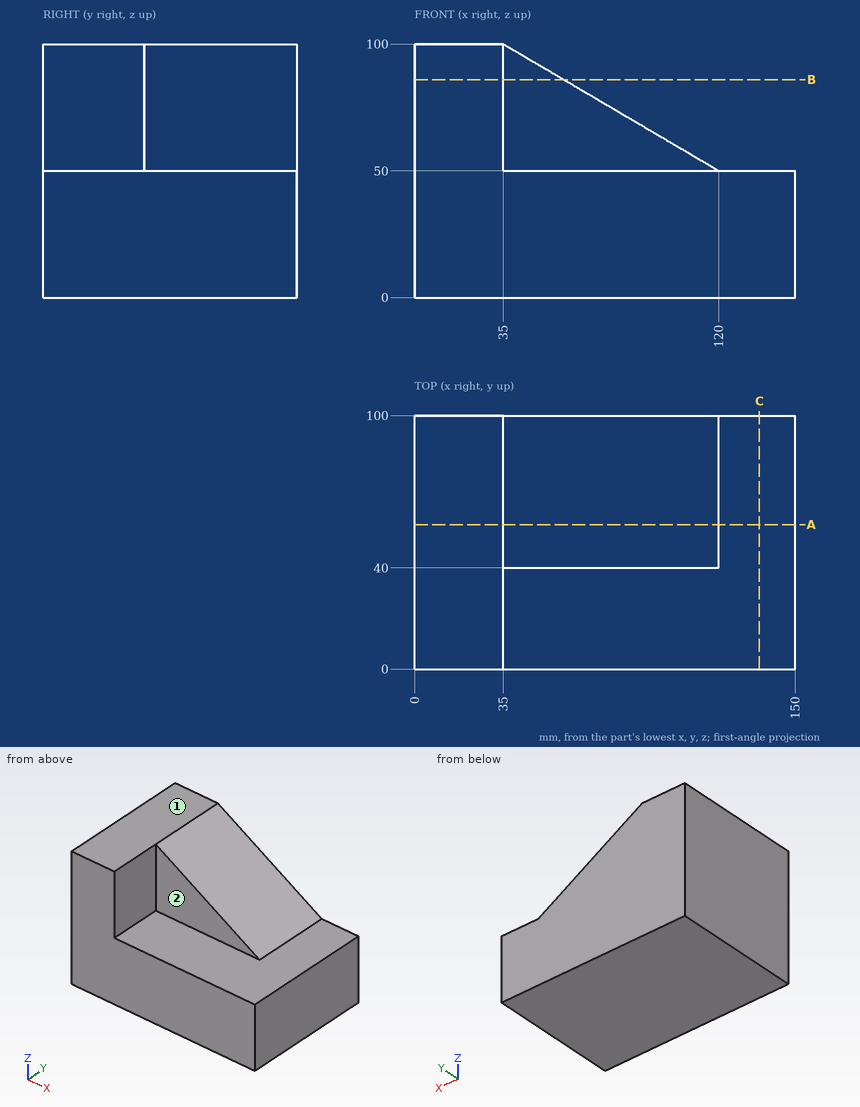
The drawing under review shows one solid part. Ordinate dimensions are in mm from its lowest x, y, z. A direction names the side the tool comes from. Round coordinates to 2 decimals unless told otherwise and drop trailing zeros. Loops run counter-clockwise (first coordinate to the right, second up) from the corner with the lowest first, then second, coordinate; pieces in that order, holes last. Notation, with made-up numbers: (-40, 71) -> (-25, 71) arc R15 ccw to (-25, 86) -> close; hole circle Ø9 at (-8.5, 25.25). An arc over 180 degrees is marked (long way). Answer in a Markdown table with one row per item.
1) Consider section C-C, the plane x = 136. Write out the cut boundary in (y, z), plus the area to 3 significant figures.
Taken from the geometry:
| item | result |
|---|---|
| outline | (0, 0) -> (100, 0) -> (100, 50) -> (0, 50) -> close |
| area | 5,000 mm² |
2) Wall thickness on line 1 along Z through (x, y) = (52.5, 37.5); line 2 along Y through (x, z) = (40, 78.5); line 3 along X through (y, z) = (12, 94.5): over which ranges is each line inside the solid? List them lowest first.
Taken from the geometry:
| item | result |
|---|---|
| line 1 | z = 0 to 50 |
| line 2 | y = 40 to 100 |
| line 3 | x = 0 to 35 |
3) Tool access review of the marked faces 1 and 2: name each direction out of +Z, -Z, +X, -X, +Y, -Y from which nothing blocks a thin tool from reaching the whole face with its end or side.
Taken from the geometry:
| item | result |
|---|---|
| face 1 | +Z, +X, -X, +Y, -Y |
| face 2 | +Z, +X, -Y |
4) Consider section B-B, the plane z = 86. Write out the cut boundary in (x, y).
Taken from the geometry:
| item | result |
|---|---|
| outline | (0, 0) -> (35, 0) -> (35, 40) -> (58.8, 40) -> (58.8, 100) -> (0, 100) -> close |
5) For pin 1 Ø1 at (x, y) = (123.5, 53.5) entering from -Z; pin 2 Ø12 at (y, z) = (11, 68) entering from +X; pin 3 Ø4 at (x, y) = (112.5, 78.5) entering from +Z; pin 4 Ø25 at (x, z) = (76, 64.5) entering from -Y, all flat-tipped, find the tip position at first contact; note any pin that passes through.
Taken from the geometry:
| item | result |
|---|---|
| pin 1 | stops at z = 0 |
| pin 2 | stops at x = 35 |
| pin 3 | stops at z = 55.59 |
| pin 4 | stops at y = 40 |
6) Consider section A-A, the plane y = 57. Write out the cut boundary in (x, z), plus the area to 3 significant figures.
Taken from the geometry:
| item | result |
|---|---|
| outline | (0, 0) -> (150, 0) -> (150, 50) -> (120, 50) -> (35, 100) -> (0, 100) -> close |
| area | 11,400 mm² |
